Part model, mm, in its own coordinate system. Round coordinates to 2 decimals unless told otherwise and drop trailing zeros. Order: outer loops, then holes, each group sorted by start corner. A loop starts at its lowest first (then second) coordinate and runs counter-clockwise, first axis right, second up. Notation, with made-up numbers: M -7.75,55.5 L 11.25,55.5 A16 cw 11.25,84.5 Z; hole C -25.5,-13 d7. An arc over 180 degrees is marked long. One line per question, with ' | ' between items.
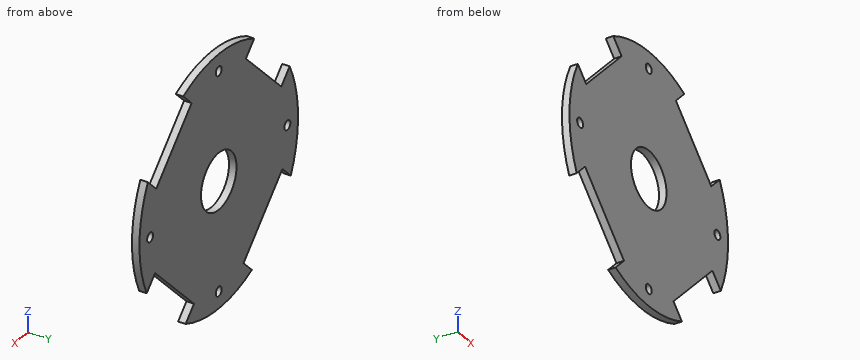
from build123d import *

# Parameters (mm, degrees)
SKETCH1_R           = 67
SKETCH1_R_2         = 2.5
BOSS_EXTRUDE1_DEPTH = 4
SKETCH2_R           = 15
CUT_EXTRUDE1_DEPTH  = 4
CUT_EXTRUDE2_DEPTH  = 10


with BuildPart() as part:
    # Sketch1 → Boss-Extrude1 (new body)
    with BuildSketch(Plane(origin=(0, 0, 0), x_dir=(1, 0, 0), z_dir=(0, 1, 0))):
        with Locations(Location((0, 0, 0), (0, 0, 270))):
            Circle(SKETCH1_R)
        with Locations(Location((-58, 0, 0), (0, 0, 270))):
            Circle(SKETCH1_R_2, mode=Mode.SUBTRACT)
        with Locations(Location((0, -58, 0), (0, 0, 270))):
            Circle(SKETCH1_R_2, mode=Mode.SUBTRACT)
        with Locations(Location((58, 0, 0), (0, 0, 270))):
            Circle(SKETCH1_R_2, mode=Mode.SUBTRACT)
        with Locations(Location((0, 58, 0), (0, 0, 270))):
            Circle(SKETCH1_R_2, mode=Mode.SUBTRACT)
    extrude(amount=BOSS_EXTRUDE1_DEPTH)

    # Sketch2 → Cut-Extrude1 (cut)
    with BuildSketch(Plane(origin=(0, 4, 0), x_dir=(1, 0, 0), z_dir=(0, 1, 0))):
        with Locations(Location((0, 0, 0), (0, 0, 270))):
            Circle(SKETCH2_R)
    extrude(amount=-CUT_EXTRUDE1_DEPTH, mode=Mode.SUBTRACT)

    # Sketch4 → Cut-Extrude2 (cut)
    with BuildSketch(Plane.XZ):
        with BuildLine():
            Line((59.908263203, 30), (52.837195391, 22.928932188))
            Line((52.837195391, 22.928932188), (22.928932188, 52.837195391))
            Line((22.928932188, 52.837195391), (30, 59.908263203))
            ThreePointArc((30, 59.908263203), (47.376154339, 47.376154339), (59.908263203, 30))
        make_face()
        with BuildLine():
            Line((-59.908263203, 30), (-52.837195391, 22.928932188))
            Line((-52.837195391, 22.928932188), (-22.928932188, 52.837195391))
            Line((-22.928932188, 52.837195391), (-30, 59.908263203))
            ThreePointArc((-30, 59.908263203), (-47.376154339, 47.376154339), (-59.908263203, 30))
        make_face()
        with BuildLine():
            Line((-53.797643362, -20.928932188), (-20.928932188, -53.797643362))
            Line((-20.928932188, -53.797643362), (-28, -60.868711174))
            ThreePointArc((-28, -60.868711174), (-47.376154339, -47.376154339), (-60.868711174, -28))
            Line((-60.868711174, -28), (-53.797643362, -20.928932188))
        make_face()
        with BuildLine():
            Line((53.797643362, -20.928932188), (20.928932188, -53.797643362))
            Line((20.928932188, -53.797643362), (28, -60.868711174))
            ThreePointArc((28, -60.868711174), (47.376154339, -47.376154339), (60.868711174, -28))
            Line((60.868711174, -28), (53.797643362, -20.928932188))
        make_face()
    extrude(amount=-CUT_EXTRUDE2_DEPTH, mode=Mode.SUBTRACT)


solid = part.part
1) Saw through at D-D (z = 27.5). List the corners of the cut face in (x, y), plus the area to 3 significant figures.
The answers:
outline: M -61.1,0 L -57.41,0 L -57.41,4 L -61.1,4 Z; M -48.27,0 L 48.27,0 L 48.27,4 L -48.27,4 Z; M 57.41,0 L 61.1,0 L 61.1,4 L 57.41,4 Z | area: 416 mm²
2) Probe line 1 (X direction, y = 2, z = 0); line 2 (Z direction, x = 25, y = 2.55); line 3 (X direction, y = 3.75, z = 1). List the from-to ranges inside material, lowest first. Write a range as [from, to].
The answers:
line 1: x = [-67, -60.5], [-55.5, -15], [15, 55.5], [60.5, 67] | line 2: z = [-62.16, -57.87], [-49.73, 50.77], [54.91, 62.16] | line 3: x = [-66.99, -60.29], [-55.71, -14.97], [14.97, 55.71], [60.29, 66.99]
3) Saw through at A-A (z = 0). List the corners of the cut face in (x, y).
The answers:
outline: M -67,0 L -60.5,0 L -60.5,4 L -67,4 Z; M -55.5,0 L -15,0 L -15,4 L -55.5,4 Z; M 15,0 L 55.5,0 L 55.5,4 L 15,4 Z; M 60.5,0 L 67,0 L 67,4 L 60.5,4 Z
4) Drop flat-ended pins along their axis: pin 1 (1 mm diameter, centred on y = 1, z = 19.5, fed in from +X); pin 2 (1 mm diameter, centred on x = -21, y = 2.5, fed in from -Z); pin 3 (4.5 mm diameter, centred on x = -58, z = 0, fed in from +Y). Give the stop position or say it passes through.
The answers:
pin 1: stops at x = 64.25 | pin 2: stops at z = -63.79 | pin 3: passes through
5) Saw through at C-C (x = 58). List the corners of the cut face in (y, z).
The answers:
outline: M 0,-25.13 L 4,-25.13 L 4,-2.5 L 0,-2.5 Z; M 0,2.5 L 4,2.5 L 4,28.09 L 0,28.09 Z
6) Saw through at B-B (y = 0.9). List the corners of the cut face in (x, z), plus the area to 3 significant figures.
The answers:
outline: M -60.87,-28 L -53.8,-20.93 L -20.93,-53.8 L -28,-60.87 A67 ccw 28,-60.87 L 20.93,-53.8 L 53.8,-20.93 L 60.87,-28 A67 ccw 59.91,30 L 52.84,22.93 L 22.93,52.84 L 30,59.91 A67 ccw -30,59.91 L -22.93,52.84 L -52.84,22.93 L -59.91,30 A67 ccw Z; hole C -58,0 d5; hole C 0,0 d30; hole C 0,-58 d5; hole C 0,58 d5; hole C 58,0 d5 | area: 11,100 mm²
